Solid Edge part; units mm, degrees
sketch "Sketch1" plane through (0, 0, 0) normal (0, -1, 0) x (1, 0, 0)
  line L0 (50, 50) -> (-50, 50)
  line L1 (-50, 50) -> (-50, -50)
  line L2 (-50, -50) -> (50, -50)
  line L3 (50, -50) -> (50, 50)
  dimension "D1" = 50
  dimension "D2" = 50
extrude "Protrusion1" add sketch "Sketch1" against normal blind 100
shell "Thinwall1" thickness 3 removed faces 3 at (-32.3333, 0, 34.3333) at (34.3333, 82.3333, 50) at (50, 82.3333, -34.3333)
Geometry: final body of the model. Coordinates: model frame, mm. A direction names the side the tool comes from. Coordinates: 2 decimals unless noted, no trailing zeros. Loops run counter-clockwise (first coordinate to the right, second up) from the corner with the lowest first, then second, coordinate; pieces in that order, holes last. Notation, with made-up numbers: M -7,69.5 L 17,69.5 A17 ccw 17,79.5 Z; hole C 13,48.5 d7. An arc over 180 degrees is marked long. Put each result on its own line as item: value.
(1) Material intervals for probe 1 along Y at (x, z) = (18.5, 13.5); probe 2 along Z at (x, y) = (13.5, 73), sorted ascending.
Answer sheet:
probe 1: y = 97 to 100
probe 2: z = -50 to -47
(2) First-contact query: pin 1 (1 mm diameter, centred on x = 17, z = 40, fed in from -Y); pin 2 (8 mm diameter, centred on y = 45, z = -4, fed in from +X). Flat tips, straight axial feed; report the tip coordinate or a pass-through.
Answer sheet:
pin 1: stops at y = 97
pin 2: stops at x = -47
(3) Cut plane A-A on y = 13.5. Return the cut outline in (x, z), then the cut area to 3 significant figures.
Answer sheet:
outline: M -50,-50 L 50,-50 L 50,-47 L -47,-47 L -47,50 L -50,50 Z
area: 591 mm^2
(4) Access query for faces 4 (the face through (2, 97, 2)), 5 (the face through (-22, 0, -48)). Directions: +Z, -Z, +X, -X, +Y, -Y. A direction counts if a zero-diameter tool reaches every point of the face in a straight line with its end or side. Return the directions, or none.
Answer sheet:
face 4: +Z, +X, -Y
face 5: +Z, -Z, +X, -X, -Y
(5) Cut plane B-B on z = -34. Return the cut outline in (x, y), then the cut area to 3 significant figures.
Answer sheet:
outline: M -50,0 L -47,0 L -47,97 L 50,97 L 50,100 L -50,100 Z
area: 591 mm^2
(6) Draft query along X for faces 1 (the face through (50, 72, -48)), 2 (the face through (-50, 49, 1)), 3 (the face through (1, 48, -47)). Return one class per face: pulls with the +X half, pulls with the -X half, needs draft (parallel to the pull), parting line crosses it, or undercut.
Answer sheet:
face 1: pulls with the +X half
face 2: pulls with the -X half
face 3: needs draft
